Work out the finished part from the listing and answer in its coordinate system (mm). Face numbers are marked on the shaded views. A direction names the side the tool comes from. Round coordinates to 2 decimals unless told otherwise and drop trailing zeros. Write each loop counter-clockwise with the first axis right and the second up, starting at its lowest first coordinate (ties: lowest second). Pieces come first, ordered by that corner, then holes.
1. A tool of negligible diameter and unlimited length cuts with its end or side. For the marked faces 4, 5 and 6, from which of +Z, -Z, +X, -X, +Y, -Y can it reach the whole face along a straight path? Write none if from no direction.
2. Determine the mould class of the marked faces 1, 2 and 3 for opening direction Y: pulls with the +Y half, pulls with the -Y half, needs draft (parallel to the pull), parting line crosses it, or undercut.
3. Find section A-A (z = 2.75). Write down the section's boundary in (x, y).
4. Find section D-D (y = 9.5). Write down the section's boundary in (x, z), and give its area (3 significant figures).
5. Find section C-C (x = 10). Write down the section's boundary in (y, z), and give its area (3 significant figures).
6. Straight lines are drawn through the part: probe 1 along X at (y, z) = (1.5, 5.75); probe 2 along Z at (x, y) = (-7.5, 4.5); probe 3 along Y at (x, z) = (3.5, 9). For each, find the intervals that lie inside material, in ascending order.
7. Flat-ended cylindrical pins translate along their axes: pin 1 Ø8 at (y, z) = (-6.5, 6) entering from -X; pin 2 Ø3 at (y, z) = (6, 2.5) entering from +X; pin 3 Ø10 at (y, z) = (-5.5, 4) entering from -X. Find the tip coordinate at first contact, or state that the pin passes through.
Autodesk Inventor part; units mm, degrees
ref_plane "Arbeitsebene1" through (16.5, 0, 0) normal (1, 0, 0) x (0, 1, 0)
ref_plane "Arbeitsebene2" through (0, 0, 13.9) normal (0, 0, 1) x (1, 0, 0)
ref_plane "XZ Plane" through (0, 0, 0) normal (0, 1, 0) x (-1, 0, 0)
sketch "Skizze1" plane through (0, 0, 0) normal (0, 0, 1) x (1, 0, 0)
  circle A0 centre (0, 0) radius 16
  circle A1 centre (-3.5, 0) radius 3
  circle A2 centre (3.5, 0) radius 2
  line L0 (-22.4, 0) -> (22.4, 0) construction
  line L1 (0, -22.4) -> (0, 22.4) construction
  circle A3 centre (0, 0) radius 3.5 construction
  dimension "d0" = 32
  dimension "d3" = 6
  dimension "d4" = 4
  dimension "d5" = 3.5
  dimension "d6" = 3.5
  dimension "d7" = 7
extrude "Extrusion1" add sketch "Skizze1" along normal blind 3.6
sketch "Skizze2" plane through (0, 0, 3.6) normal (0, 0, 1) x (1, 0, 0)
  circle A0 centre (0, 0) radius 16
  circle A1 centre (-3.5, 0) radius 3
  circle A2 centre (-3.5, 0) radius 3
  circle A3 centre (3.5, 0) radius 2
  circle A4 centre (3.5, 0) radius 2
  circle A5 centre (0, 0) radius 7.8
  circle A6 centre (0, 0) radius 13.75
  dimension "d10" = 15.6
  dimension "d11" = 27.5
  dimension "d12" = 4
  dimension "d13" = 32
  dimension "d14" = 6
extrude "Extrusion2" add sketch "Skizze2" along normal blind 5.8
sketch "Skizze4" plane through (0, 0, 0) normal (0, 0, -1) x (-1, 0, 0)
  circle A0 centre (0, 0) radius 7.8 construction
  circle A1 centre (3.5, 0) radius 3 construction
  circle A2 centre (-3.5, 0) radius 2 construction
  circle A3 centre (0, 0) radius 7
  dimension "d29" = 14
extrude "Extrusion4" cut sketch "Skizze4" against normal blind 8
sketch "Skizze5" plane through (0, 0, 8) normal (0, 0, -1) x (-1, 0, 0)
  circle A0 centre (-3.5, 0) radius 2 construction
  line L0 (-1.5, 0) -> (0.5, 0) construction
  circle A1 centre (3.5, 0) radius 3 construction
  line L1 (-0.5, -6.9821) -> (-0.5, 6.9821) construction
  circle A2 centre (0, 0) radius 7 construction
  circle A3 centre (0, 0) radius 7
  arc A4 (3.2508, 6.1994) -> (3.1701, -6.241) centre (7.631, -0.0495) ccw
  arc A5 (2.3003, 6.6112) -> (2.2144, -6.6405) centre (7.631, -0.0495) ccw
  point P0 (0.1, -6.9993)
  point P1 (0.1, 6.9993)
  point P2 (-1.1, -6.913)
  point P3 (-1.1, 6.913)
  dimension "d35" = 0
  dimension "d39" = 8.5312
  dimension "d40" = 7.6312
  dimension "d41" = 4
  dimension "d42" = 8.1311
  dimension "d43" = 0.0495
  dimension "d44" = 0.6
  dimension "d45" = 0.6
  dimension "d46" = 0.6
  dimension "d47" = 0.6
extrude "Extrusion5" add sketch "Skizze5" along normal blind 8 contours A4 A3 A5
sketch "Skizze6" plane through (0, 0, 3.6) normal (0, 0, 1) x (1, 0, 0)
  circle A0 centre (0, 0) radius 7.8
  circle A1 centre (0, 0) radius 13.75
extrude "Extrusion6" cut sketch "Skizze6" against normal blind 1.6
sketch "Skizze7" plane through (0, 0, 0) normal (0, 0, -1) x (-1, 0, 0)
  circle A0 centre (0, 0) radius 16
  line L0 (0, 16) -> (0, 14.8) construction
  line L1 (0, 16) -> (1.2, 16) construction
  line L2 (0, 14.8) -> (-6.0795, 14.8)
  line L3 (0, 14.8) -> (6.0795, 14.8) construction
  line L4 (0, 14.8) -> (6.0795, 14.8)
  line L5 (0, 14.8) -> (6.0795, 14.8) construction
  point P0 (-0.8, 15.98)
  point P1 (0.8, 15.98)
  point P2 (0, 15.4)
  dimension "d50" = 1.2
  dimension "d51" = 90
  dimension "d70" = 1.18
  dimension "d71" = 1.18
extrude "Extrusion7" cut sketch "Skizze7" against normal blind 5 contours L4 L2 A0 picked at (-3.0593, 15.099)
sketch "Skizze8" plane through (0, 0, 9.4) normal (0, 0, 1) x (1, 0, 0)
  circle A0 centre (0, 0) radius 13.75
  circle A1 centre (0, 0) radius 16
  dimension "d55" = 27.5
  dimension "d56" = 32
extrude "Extrusion8" add sketch "Skizze8" along normal blind 8
ref_plane "Arbeitsebene1" through (16.5, 0, 0) normal (1, 0, 0) x (0, 1, 0)
sketch "Skizze9" plane through (16.5, 0, 0) normal (1, 0, 0) x (0, 1, 0)
  point P0 (0, 0)
  point P1 (0, 14)
  dimension "d67" = 14
hole "Bohrung1" at (16.5, 0, 14) direction (-1, 0, 0) diameter 3 depth 3.25
sketch "Skizze10" plane through (0, 0, 0) normal (1, 0, 0) x (0, 1, 0)
  line L0 (14.8, 5) -> (14.8, 0)
  line L1 (14.8, 5) -> (16.0125, 6.2125)
  line L2 (14.8, 5) -> (16.5147, 5) construction
  line L3 (16.0125, 6.2125) -> (16.1276, 4.8849)
  line L4 (16.1276, 4.8849) -> (14.8, 5)
  point P0 (0, 0)
  dimension "d72" = 45
  dimension "d73" = 4.955
  dimension "d74" = 85.045
  dimension "d75" = 1.3127
extrude "Extrusion9" cut sketch "Skizze10" against normal mid plane 29.25
ref_plane "Arbeitsebene2" through (0, 0, 13.9) normal (0, 0, 1) x (1, 0, 0)
sketch "Skizze11" plane through (0, 0, 13.9) normal (0, 0, 1) x (1, 0, 0)
  line L0 (13.6679, 1.5) -> (15.9295, 1.5) construction
  line L1 (13.6679, -1.5) -> (15.9295, -1.5) construction
  arc A0 (14.2726, -2.5) -> (14.2726, 2.5) centre (0, 0) ccw
  arc A1 (13.146, -2.5) -> (13.146, 2.5) centre (0, 0) ccw
  line L2 (14.2726, 2.5) -> (13.146, 2.5)
  line L3 (13.3816, 0) -> (15.9295, 0) construction
  line L4 (14.2726, -2.5) -> (13.146, -2.5)
  dimension "d79" = 14.4899
  dimension "d80" = 13.3816
  dimension "d81" = 4
  dimension "d82" = 1.5
extrude "Extrusion10" cut sketch "Skizze11" along normal blind 3.75 and the other way blind 2
chamfer "Fase3" distance 0.6 angle 45 1 edges at (14.4899, 0, 11.9)
chamfer "Fase4" distance 0.1398 angle 45 2 edges at (13.6926, -1.2552, 11.9) (13.6926, 1.2552, 11.9)
chamfer "Fase5" distance 0.751 angle 45 2 edges at (14.2726, 2.5, 14.95) (14.2726, -2.5, 14.95)
properties part number "Bottom" material "PC/ABS-Kunststoff"
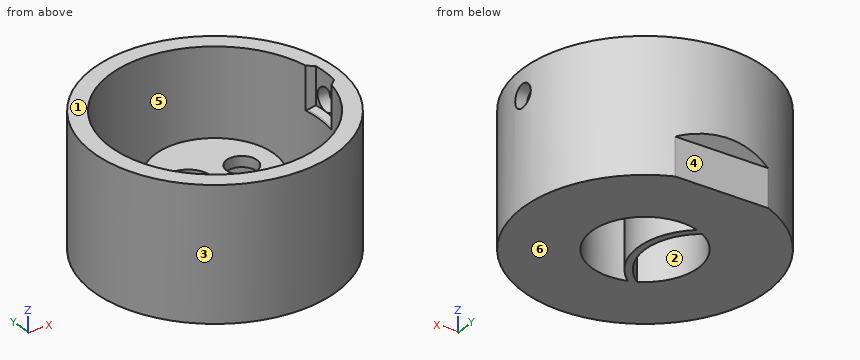
Worked answers:
1. face 4: -Z, +X, -X, +Y
1. face 5: +Z
1. face 6: -Z, +X, -X, +Y, -Y
2. face 1: needs draft
2. face 2: undercut
2. face 3: parting line crosses it
3. outline: circle Ø15.6 at (0, 0); (-6.08, 14.8) arc R16 ccw (long way) to (6.08, 14.8) - close; hole circle Ø27.5 at (0, 0); hole (-3.25, 6.2) arc R7 ccw to (-3.17, -6.24) arc R7.63 ccw to start; hole (-2.3, 6.61) arc R8.53 cw to (-2.21, -6.64) arc R7 ccw (long way) to start
4. outline: (-12.87, 0) - (12.87, 0) - (12.87, 17.4) - (9.94, 17.4) - (9.94, 2) - (-9.94, 2) - (-9.94, 17.4) - (-12.87, 17.4) - close
4. area: 142 mm2
5. outline: (-12.49, 0) - (12.49, 0) - (12.49, 17.4) - (9.44, 17.4) - (9.44, 2) - (-9.44, 2) - (-9.44, 17.4) - (-12.49, 17.4) - close
5. area: 144 mm2
6. probe 1: x = -15.93 to -13.67, -7.65 to -6.84, -0.16 to 0.76, 6.84 to 7.65, 13.67 to 15.93
6. probe 2: z = 0 to 2
6. probe 3: y = -15.61 to -13.3, -6.97 to -2, 2 to 6.97, 13.3 to 15.61
7. pin 1: stops at x = -15.8
7. pin 2: stops at x = 15.35
7. pin 3: stops at x = -15.99
